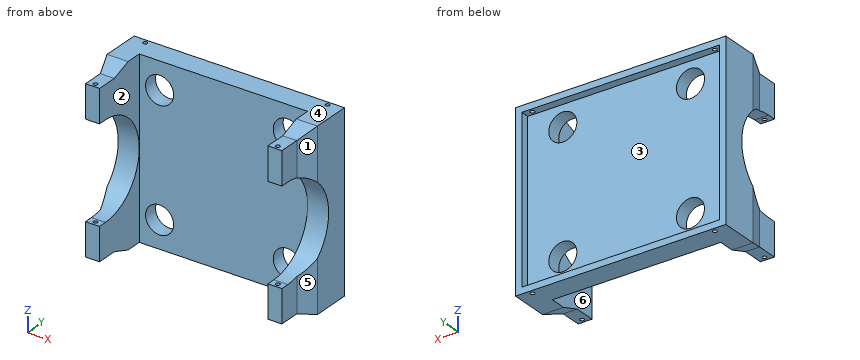
Autodesk Inventor part; units mm, degrees
ref_plane "YZ Plane" through (0, 0, 0) normal (1, 0, 0) x (0, 1, 0)
ref_plane "XZ Plane" through (0, 0, 0) normal (0, 1, 0) x (-1, 0, 0)
ref_plane "XY Plane" through (0, 0, 0) normal (0, 0, 1) x (1, 0, 0)
sketch "스케치1" plane through (0, 0, 0) normal (0, 0, 1) x (1, 0, 0)
  line L0 (0, 0) -> (15, 0)
  line L1 (15, 0) -> (15, 40)
  line L2 (15, 40) -> (135, 40)
  line L3 (135, 40) -> (135, 0)
  line L4 (135, 0) -> (150, 0)
  line L5 (150, 0) -> (150, 50)
  line L6 (150, 50) -> (0, 50)
  line L7 (0, 50) -> (0, 0)
  line L8 (0, 28.7374) -> (5, 15)
  line L9 (5, 15) -> (5, 0)
  line L10 (75, 50) -> (75, 45.4681)
  line L11 (150, 28.7374) -> (145, 15)
  line L12 (145, 15) -> (145, 0)
  point P0 (145, 0)
  dimension "d0" = 150
  dimension "d1" = 15
  dimension "d2" = 15
  dimension "d3" = 10
  dimension "d4" = 50
  dimension "d7" = 10
  dimension "d8" = 160
  dimension "d9" = 15
extrude "돌출1" add sketch "스케치1" along normal blind 125 contours L9 L8 L7 L6 L5 L11 L12 L4 L3 L2 L1 L0
sketch "스케치2" plane through (0, 28.7374, 0) normal (-1, 0, 0) x (0, 0, 1)
  line L0 (0, 21.2626) -> (125, 21.2626)
  line L1 (62.5, 21.2626) -> (62.5, 15.0045)
  line L2 (0, 0) -> (0, -13.7374)
  line L3 (0, 0) -> (5, -13.7374)
  line L4 (5, -13.7374) -> (5, -28.7374)
  line L5 (0, -28.7374) -> (125, -28.7374)
  line L6 (0, 11.2626) -> (0, -28.7374)
  line L7 (0, -28.7374) -> (0, 11.2626)
  line L8 (0, -13.7374) -> (0, -28.7374)
  line L9 (0, 0) -> (0, -13.7374)
  line L10 (0, 21.2626) -> (0, 0)
  line L11 (0, 0) -> (0, 21.2626)
  line L12 (0, -13.7374) -> (0, 0)
  line L13 (0, -28.7374) -> (0, -13.7374)
  line L14 (125, -28.7374) -> (125, -13.7374)
  line L15 (125, -13.7374) -> (125, 0)
  line L16 (125, 0) -> (125, 21.2626)
  line L17 (125, 21.2626) -> (125, 0)
  line L18 (125, 0) -> (125, -13.7374)
  line L19 (125, -13.7374) -> (125, -28.7374)
  line L20 (125, -28.7374) -> (125, 11.2626)
  line L21 (125, 11.2626) -> (125, -28.7374)
  line L22 (125, 0) -> (120, -13.7374)
  line L23 (120, -13.7374) -> (120, -28.7374)
  dimension "d10" = 15
  dimension "d11" = 160
extrude "돌출2" cut sketch "스케치2" against normal through all contours L3 L4 L5 L6 L2 | L15 L14 L5 L23 L22
sketch "스케치3" plane through (0, 50, 0) normal (0, 1, 0) x (1, 0, 0)
  line L0 (150, 0) -> (0, 0)
  line L1 (0, 0) -> (0, -125)
  line L2 (150, -125) -> (0, -125)
  line L3 (150, 0) -> (150, -125)
  line L4 (4.5, -4.5) -> (145.5, -4.5)
  line L5 (145.5, -4.5) -> (145.5, -120.5)
  line L6 (145.5, -120.5) -> (4.5, -120.5)
  line L7 (4.5, -120.5) -> (4.5, -4.5)
  circle A0 centre (29.5, -19.5) radius 10
  circle A1 centre (29.5, -105.5) radius 10
  circle A2 centre (120.5, -19.5) radius 10
  circle A3 centre (120.5, -105.5) radius 10
  point P0 (0, 0)
  dimension "d14" = 4.5
  dimension "d17" = 20
  dimension "d18" = 15
  dimension "d19" = 25
  dimension "d20" = 25
  dimension "d21" = 15
extrude "돌출3" add sketch "스케치3" along normal blind 6 contours L3 L2 L1 L0
extrude "돌출4" cut sketch "스케치3" against normal through all contours A0 | A1 | A2 | A3
sketch "스케치5" plane through (0, 0, 0) normal (0, 0, -1) x (-1, 0, 0)
  circle A0 centre (-140, 53) radius 1.5
  line L0 (-135, 0) -> (-145, 0)
  line L1 (-150, 56) -> (0, 56)
  line L2 (-4.5, 56) -> (-145.5, 56)
  line L3 (-75, 56) -> (-75, 53)
  circle A1 centre (-10, 53) radius 1.5
  circle A2 centre (-140, 3) radius 1.5
  circle A3 centre (-10, 3) radius 1.5
  point P0 (0, 0)
  point P1 (-140, 0)
  dimension "d30" = 3
  dimension "d31" = 3
  dimension "d34" = 3
extrude "돌출6" cut sketch "스케치5" against normal through all
sketch "스케치6" plane through (0, 28.7374, 0) normal (-1, 0, 0) x (0, 0, 1)
  arc A0 (96.5, -22.7374) -> (28.5, -22.7374) centre (62.5, -22.7374) ccw
  line L0 (5, -28.7374) -> (120, -28.7374)
  line L1 (28.5, -22.7374) -> (28.5, -28.7374)
  line L2 (96.5, -28.7374) -> (96.5, -22.7374)
  point P0 (0, -28.7374)
  point P1 (62.5, -28.7374)
  point P2 (99.6652, -28.7374)
  point P3 (25.3348, -28.7374)
  dimension "d35" = 68
  dimension "d38" = 6
extrude "돌출7" cut sketch "스케치6" against normal through all
equation "\"d10\" = d9"
equation "\"d11\" = d8"
equation "\"d20\" = d19"
equation "\"d21\" = d18"
equation "\"d34\" = d30"
properties part number "partContainer"
CAD build for the part. Positions are in the model's coordinates, mm. Face numbers are marked on the shaded views. A direction names the side the tool comes from. Round coordinates to 2 decimals unless told otherwise and drop trailing zeros. Loops run counter-clockwise (first coordinate to the right, second up) from the corner with the lowest first, then second, coordinate; pieces in that order, holes last. Notation, with made-up numbers: M 46,17 L 87,17 A20 cw 87,23 Z; hole C 25,27 d4. An arc over 180 degrees is marked long. Use a Markdown table: item, result. Add a question column.
(1) Cut at A-A (x = 37.5). Give the cut face in (y, z).
(2) Pull direction X, two halves, no side cores. Call the marked faces 4, 5 and 6: +X half, -X half, draft (parallel to the pull), parting line (faces both ways), or undercut.
(3) Cut at C-C (y = 12). Give the cut face in (x, z).
(4) Flat gauge pins, fed straight in: pin 1 (23 mm diameter, centred on x = 29.5, z = 19.5, fed in from +Y); pin 2 (4 mm diameter, centred on x = 10, y = 3, fed in from +Z); pin 3 (5 mm diameter, centred on x = 139, y = 6, fed in from -Z). Where does each tip first touch, or does it go through?
(5) Drill centre lines: line 1 (X direction, y = 47, z = 19); line 2 (Z direction, x = 29.5, y = 43.75); line 3 (Z direction, x = 123, y = 50.5). Where is each one in solid material? Low to high.
(6) Which spindle directions (+Z, -Z, +X, -X, +Y, -Y) get a long thin tool onto all of the face, cutting with end or side? Do the marked faces 1, 2 and 3. Say none if no direction does.
(7) Cut at B-B (z = 21.5). Give the cut face in (x, y).
(8) Cut at D-D (x = 54). Give the cut face in (y, z).
Geometry says:
| question | item | result |
|---|---|---|
| 1 | outline | M 40,0 L 56,0 L 56,4.5 L 50,4.5 L 50,13.5 L 40,13.5 Z; M 40,25.5 L 50,25.5 L 50,99.5 L 40,99.5 Z; M 40,111.5 L 50,111.5 L 50,120.5 L 56,120.5 L 56,125 L 40,125 Z |
| 2 | face 4 | draft |
| 2 | face 5 | +X half |
| 2 | face 6 | undercut |
| 3 | outline | M 5,5 L 15,5 L 15,29.03 L 5,29.03 Z; M 5,95.97 L 15,95.97 L 15,120 L 5,120 Z; M 135,5 L 145,5 L 145,29.03 L 135,29.03 Z; M 135,95.97 L 145,95.97 L 145,120 L 135,120 Z |
| 4 | pin 1 | stops at y = 50 |
| 4 | pin 2 | stops at z = 120 |
| 4 | pin 3 | stops at z = 5 |
| 5 | line 1 | x = 0 to 19.51, 39.49 to 110.51, 130.49 to 150 |
| 5 | line 2 | z = 0 to 9.5, 29.5 to 95.5, 115.5 to 125 |
| 5 | line 3 | z = 0 to 4.5, 120.5 to 125 |
| 6 | face 1 | +Z, -Z, +X, -Y |
| 6 | face 2 | +Z, -Z, -Y |
| 6 | face 3 | +Y |
| 7 | outline | M 0,28.74 L 5,15 L 5,0 L 15,0 L 15,40 L 19.7,40 L 19.7,50 L 4.5,50 L 4.5,56 L 0,56 Z; M 39.3,40 L 110.7,40 L 110.7,50 L 39.3,50 Z; M 130.3,40 L 135,40 L 135,0 L 145,0 L 145,15 L 150,28.74 L 150,56 L 145.5,56 L 145.5,50 L 130.3,50 Z; hole C 10,3 d3; hole C 140,3 d3 |
| 8 | outline | M 40,0 L 56,0 L 56,4.5 L 50,4.5 L 50,120.5 L 56,120.5 L 56,125 L 40,125 Z |
